Here's the drawing with two shaded views (mm, measured from the low corner). I have some questions. Coordinates: 2 decimals unless noted, no trailing zeros. Write each loop counter-clockwise with the first axis right and the second up, starting at its lowest first coordinate (ties: lowest second). Pieces come first, ordered by that corner, then holes. Notation, with made-up numbers: M 80.5,78.25 L 92.5,78.25 A16 ccw 92.5,109.25 Z; hole C 71.5,17.5 d4. An arc over 180 degrees is marked long. Answer as CSV lines item,"result". Start each with the question number.
Item 1: Suppose I cut it at B-B, the plane x = 132.25. Write out the boundary of the cut face in (y, z), and give its area (3 significant figures).
Item 2: Suppose I cut it at A-A, the plane z = 7.75. Write out the boundary of the cut face in (x, y).
Item 3: I'm going to push a flat-ended pin straight in: P1, Ø4, axis at x = 132.25, z = 132.25, coming from the +Y side. Where does the tip first touch, or does it pass through?
Item 4: If I drill on line 1 along X through (y, z) = (17, 7.75); line 2 along X through (y, z) = (10.75, 9.5), over which ranges is the centre line in solid material (lowest first)? Write a range as [from, to].
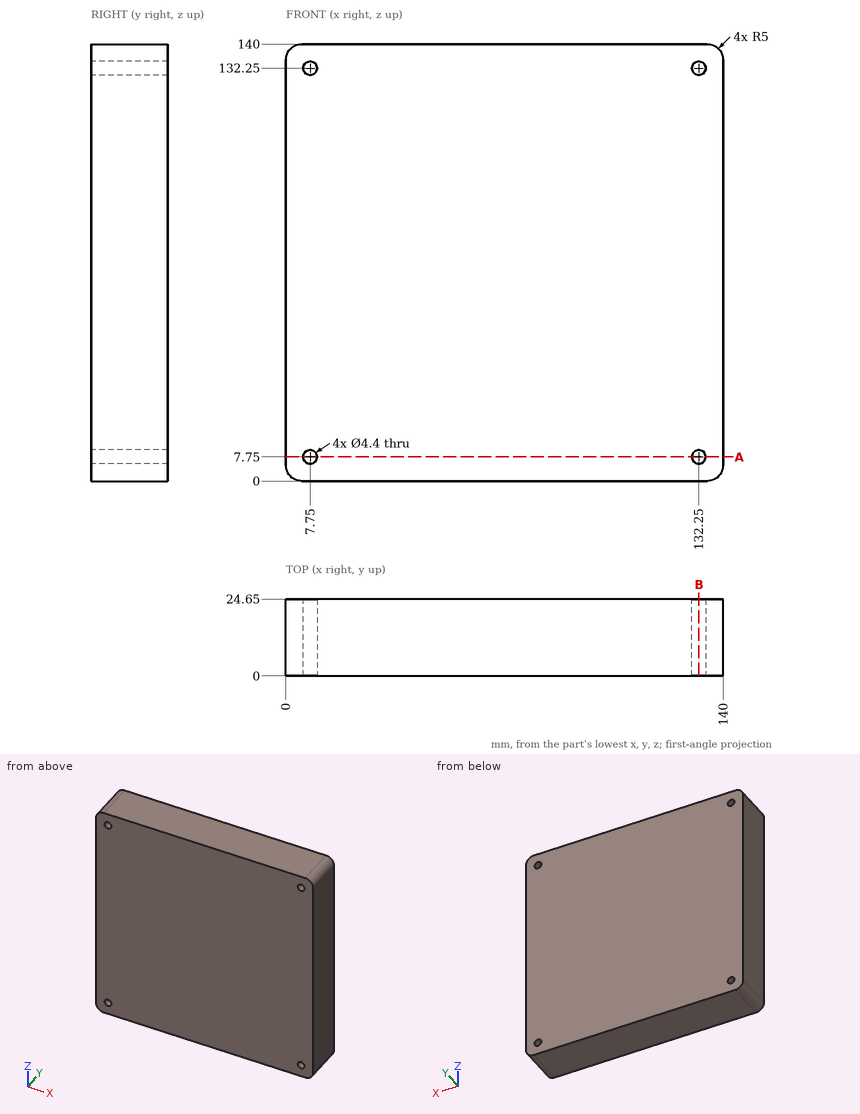
Ans:
1,outline,"M 0,0 L 24.65,0 L 24.65,5.55 L 0,5.55 Z; M 0,9.95 L 24.65,9.95 L 24.65,130.05 L 0,130.05 Z; M 0,134.45 L 24.65,134.45 L 24.65,140 L 0,140 Z"
1,area,"3,230 mm^2"
2,outline,"M 0,0 L 5.55,0 L 5.55,24.65 L 0,24.65 Z; M 9.95,0 L 130.05,0 L 130.05,24.65 L 9.95,24.65 Z; M 134.45,0 L 140,0 L 140,24.65 L 134.45,24.65 Z"
3,P1,"passes through"
4,line 1,"x = [0, 5.55], [9.95, 130.05], [134.45, 140]"
4,line 2,"x = [0, 6.42], [9.08, 130.92], [133.58, 140]"
